```python
from build123d import *

# Parameters (mm, degrees)
F0_W     = 50.8
F0_H     = 50.8
F1_DEPTH = 12.7
F2_W     = 50.8
F2_H     = 50.8
F3_DEPTH = 12.7
F4_R     = 6.35
F5_DEPTH = 25.4


with BuildPart() as f1:
    # F0 (on Front) → F1 (new body)
    with BuildSketch(Plane.XZ):
        with Locations((1.379482, -15.815881)):
            Rectangle(F0_W, F0_H)
    extrude(amount=F1_DEPTH)

    # F2 (on Top) → F3 (join)
    with BuildSketch(Plane.XY):
        with Locations((0.965637, 12.567736)):
            Rectangle(F2_W, F2_H)
    extrude(amount=F3_DEPTH)

    # F4 (on face) → F5 (cut)
    with BuildSketch(Plane.XY):
        with Locations((2.483068, 20.968137)):
            Circle(F4_R)
    extrude(amount=F5_DEPTH, mode=Mode.SUBTRACT)


solid = f1.part
```
Geometry: final body of the model. Coordinates: model frame, mm. A direction names the side the tool comes from. Round coordinates to 2 decimals unless told otherwise and drop trailing zeros. Order: outer loops, then holes, each group sorted by start corner. A loop starts at its lowest first (then second) coordinate and runs counter-clockwise, first axis right, second up. Notation, with made-up numbers: (-8.5, -37) -> (24.5, -37) arc R11 cw to (24.5, -20) -> close; hole circle Ø1 at (42, 30.5). An arc over 180 degrees is marked (long way). Use one line per item in the form item = value. Start each with the question number.
1. Reachability of faces 1 (the face through (-24.021, -6, -21)), 2 (the face through (1, -6, -41.216)) from +Z, -Z, +X, -X, +Y, -Y: full face, straight path, thin tool, end or side. Return the list, or none.
2. Cut plane A-A (y = 16.5). Return the cut outline in (x, z).
3. Cut plane C-C (x = 10). Return the cut outline in (y, z), then the cut area to 3 significant figures.
4. Line query: probe 1 along X at (y, z) = (28.5, 7.5); probe 2 along Z at (x, y) = (22.5, 4.5); probe 3 along Y at (x, z) = (14, -13). Output: solid intervals per line, ascending.
5. Cut plane D-D (z = -30). Return the cut outline in (x, y).
6. Pin query (flat end, axial travel): pin 1 Ø10 at (y, z) = (-7, -21) entering from -X; pin 2 Ø3 at (x, y) = (21.5, 9.5) entering from -Z; pin 3 Ø14 at (y, z) = (12, 5.5) entering from +X. Return the tip coordinate at first contact, or that it passes through.
7. Cut plane B-B (x = 1). Return the cut outline in (y, z).
Solution:
q1.face_1 = -Z, -X, +Y, -Y
q1.face_2 = -Z, +X, -X, +Y, -Y
q2.outline = (-24.43, 0) -> (-2.03, 0) -> (-2.03, 12.7) -> (-24.43, 12.7) -> close; (7, 0) -> (26.37, 0) -> (26.37, 12.7) -> (7, 12.7) -> close
q3.outline = (-12.83, 0) -> (-12.7, 0) -> (-12.7, -41.22) -> (0, -41.22) -> (0, 0) -> (37.97, 0) -> (37.97, 12.7) -> (-12.83, 12.7) -> close
q3.area = 1,170 mm^2
q4.probe_1 = -24.43 to 26.37
q4.probe_2 = 0 to 12.7
q4.probe_3 = -12.7 to 0
q5.outline = (-24.02, -12.7) -> (26.78, -12.7) -> (26.78, 0) -> (-24.02, 0) -> close
q6.pin_1 = -24.02
q6.pin_2 = 0
q6.pin_3 = 26.37
q7.outline = (-12.83, 0) -> (-12.7, 0) -> (-12.7, -41.22) -> (0, -41.22) -> (0, 0) -> (14.79, 0) -> (14.79, 12.7) -> (-12.83, 12.7) -> close; (27.14, 0) -> (37.97, 0) -> (37.97, 12.7) -> (27.14, 12.7) -> close
